Could you check a few things on this model? Use its own coordinates, in mm. Give positions to 0.01 mm unless a question says otherwise; leave off trailing zeros. Order: outer loops, then holes, each group sorted by start corner. A loop starts at its lowest first (then second) coordinate and runs counter-clockwise, first axis right, second up. Notation, with made-up numbers: M 21.5,-9 L 56.5,-9 A20 ccw 56.5,-1 Z; hole C 17,-18 d10. An arc over 180 degrees is marked long. Use a Markdown table: item, result. Add a question column.
Item 1: If I drill on L1, parallel to Z at x = 420, y = 6.5, over which ranges is the centre line in solid material (lowest first)? Write a range as from..to.
Item 2: I'm going to push flat-ended pins straight in: pin 1 Ø4 at (x, y) = (419, 27.5) entering from -Z; pin 2 Ø1.5 at (x, z) = (377, -34) entering from +Y. Where does each tip first touch, or does it pass through?
Item 3: Suppose I cut it at B-B on z = -49. Write out the boundary of the cut face in (x, y).
Item 4: Suppose I cut it at A-A on y = 51. Count the separate pieces of the cut face and the enclosed holes in it, plus the area to 3 significant figures.
Item 5: Suppose I cut it at C-C on x = 196. Write out the boundary of the cut face in (y, z), plus the area to 3 significant figures.
from build123d import *

# Parameters (mm, degrees)
SKETCH_1_W          = 450
SKETCH_1_H          = 60
EXTRUDE_1_DEPTH     = 3
EXTRUDE_2_DEPTH     = 3
CUT_EXTRUDE_1_DEPTH = 462.507313051


with BuildPart() as part:
    # 草图1 → 凸台-拉伸1 (new body)
    with BuildSketch(Plane(origin=(0, 0, 0), x_dir=(1, 0, 0), z_dir=(0, 1, 0))):
        with Locations((225, 30)):
            Rectangle(SKETCH_1_W, SKETCH_1_H)
    extrude(amount=EXTRUDE_1_DEPTH)

    # 草图3 → 凸台-拉伸2 (add)
    with BuildSketch(Plane.XY):
        Polygon((0, 0), (0, 83), (2.5, 83), (2.5, 3), (27.5, 3), (27.5, 83), (32.5, 83), (32.5, 3), (57.5, 3), (57.5, 83), (62.5, 83), (62.5, 3), (87.5, 3), (87.5, 83), (92.5, 83), (92.5, 3), (117.5, 3), (117.5, 83), (122.5, 83), (122.5, 3), (147.5, 3), (147.5, 83), (152.5, 83), (152.5, 3), (177.5, 3), (177.5, 83), (182.5, 83), (182.5, 3), (207.5, 3), (207.5, 83), (212.5, 83), (212.5, 3), (237.5, 3), (237.5, 83), (242.5, 83), (242.5, 3), (267.5, 3), (267.5, 83), (272.5, 83), (272.5, 3), (297.5, 3), (297.5, 83), (302.5, 83), (302.5, 3), (327.5, 3), (327.5, 83), (332.5, 83), (332.5, 3), (357.5, 3), (357.5, 83), (362.5, 83), (362.5, 3), (387.5, 3), (387.5, 83), (392.5, 83), (392.5, 3), (417.5, 3), (417.5, 83), (422.5, 83), (422.5, 3), (447.5, 3), (447.5, 83), (450, 83), (450, 3), (450, 0), align=None)
    extrude(amount=EXTRUDE_2_DEPTH)

    # 草图4 → 切除-拉伸1 (cut, through all)
    with BuildSketch(Plane.ZY):
        Polygon((3, 83), (0, 68), (0, 83), align=None)
    extrude(amount=-CUT_EXTRUDE_1_DEPTH, mode=Mode.SUBTRACT)


solid = part.part
Findings below:
| question | item | result |
|---|---|---|
| 1 | L1 | z = 0..3 |
| 2 | pin 1 | stops at z = 0 |
| 2 | pin 2 | stops at y = 3 |
| 3 | outline | M 0,0 L 450,0 L 450,3 L 0,3 Z |
| 4 | separate pieces | 16 |
| 4 | enclosed holes | 0 |
| 4 | area | 225 mm^2 |
| 5 | outline | M 0,-60 L 3,-60 L 3,3 L 0,3 Z |
| 5 | area | 189 mm^2 |
